from build123d import *

# Parameters (mm, degrees)
SKETCH1_W           = 25
SKETCH1_H           = 135
BOSS_EXTRUDE1_DEPTH = 3.175


with BuildPart() as part:
    # Sketch1 → Boss-Extrude1 (new body)
    with BuildSketch(Plane(origin=(0, 0, 0), x_dir=(1, 0, 0), z_dir=(0, 1, 0))):
        Polygon((67.674333466, 92.651811553), (67.674333466, -62.348188447), (-47.325666534, -62.348188447), (-47.325666534, -27.044565342), (-47.325666534, 92.651811553), align=None)
        with Locations((-6.586624165, 15.039519235)):
            Rectangle(SKETCH1_W, SKETCH1_H, mode=Mode.SUBTRACT)
        with BuildLine():
            Line((-34.586624165, 63.427366475), (-34.586624165, 83.427366475))
            ThreePointArc((-34.586624165, 83.427366475), (-32.086624165, 85.927366475), (-29.586624165, 83.427366475))
            Line((-29.586624165, 83.427366475), (-29.586624165, 63.427366475))
            ThreePointArc((-29.586624165, 63.427366475), (-32.086624165, 60.927366475), (-34.586624165, 63.427366475))
        make_face(mode=Mode.SUBTRACT)
        with BuildLine():
            Line((-34.586624165, 3.427366475), (-34.586624165, 23.427366475))
            ThreePointArc((-34.586624165, 23.427366475), (-32.086624165, 25.927366475), (-29.586624165, 23.427366475))
            Line((-29.586624165, 23.427366475), (-29.586624165, 3.427366475))
            ThreePointArc((-29.586624165, 3.427366475), (-32.086624165, 0.927366475), (-34.586624165, 3.427366475))
        make_face(mode=Mode.SUBTRACT)
        with BuildLine():
            Line((59.674333466, 7.651811553), (59.674333466, 27.651811553))
            ThreePointArc((59.674333466, 27.651811553), (61.674333466, 29.651811553), (63.674333466, 27.651811553))
            Line((63.674333466, 27.651811553), (63.674333466, 7.651811553))
            ThreePointArc((63.674333466, 7.651811553), (61.674333466, 5.651811553), (59.674333466, 7.651811553))
        make_face(mode=Mode.SUBTRACT)
        with BuildLine():
            Line((59.674333466, -40.348188447), (59.674333466, -20.348188447))
            ThreePointArc((59.674333466, -20.348188447), (61.674333466, -18.348188447), (63.674333466, -20.348188447))
            Line((63.674333466, -20.348188447), (63.674333466, -40.348188447))
            ThreePointArc((63.674333466, -40.348188447), (61.674333466, -42.348188447), (59.674333466, -40.348188447))
        make_face(mode=Mode.SUBTRACT)
        with BuildLine():
            Line((41.674333466, 7.651811553), (41.674333466, 27.651811553))
            ThreePointArc((41.674333466, 27.651811553), (39.674333466, 29.651811553), (37.674333466, 27.651811553))
            Line((37.674333466, 27.651811553), (37.674333466, 7.651811553))
            ThreePointArc((37.674333466, 7.651811553), (39.674333466, 5.651811553), (41.674333466, 7.651811553))
        make_face(mode=Mode.SUBTRACT)
        with BuildLine():
            Line((41.674333466, -40.348188447), (41.674333466, -20.348188447))
            ThreePointArc((41.674333466, -20.348188447), (39.674333466, -18.348188447), (37.674333466, -20.348188447))
            Line((37.674333466, -20.348188447), (37.674333466, -40.348188447))
            ThreePointArc((37.674333466, -40.348188447), (39.674333466, -42.348188447), (41.674333466, -40.348188447))
        make_face(mode=Mode.SUBTRACT)
    extrude(amount=BOSS_EXTRUDE1_DEPTH)


solid = part.part
Geometry check sheet. Reference: the model listing, model coordinates, mm. A direction names the side the tool comes from. Round coordinates to 2 decimals unless told otherwise and drop trailing zeros. Loops run counter-clockwise (first coordinate to the right, second up) from the corner with the lowest first, then second, coordinate; pieces in that order, holes last. Notation, with made-up numbers: (-3.5, 47.5) - (26.5, 47.5) arc R12 ccw to (26.5, 58.5) - close; hole circle Ø2 at (28, 62). An arc over 180 degrees is marked (long way). One line per question, with ' | ' between items. Start each with the question number.
1. Scan lines: line 1 (X direction, y = 2.95, z = -76); line 2 (X direction, y = 1.6, z = -14); line 3 (X direction, y = 1.9, z = 26). Record each from-to range of solid material in increasing order. Write a range as [from, to].
2. Tool access check on faces 1 (the face through (63.674, 2, 30)), 2 (the face through (11, 3.175, -16)). Record the directions out of +Z, -Z, +X, -X, +Y, -Y that give a thin tool (end or side, any length) a straight path to the whole face; none if there is none.
3. Cross-section at B-B on x = -7. Record the cut outline in (y, z) (3 decimals).
4. Draft check along X on faces 3 (the face through (11, 2, 62.348)), 4 (the face through (37.674, 2, -18)), 5 (the face through (-47.326, 2, -16)). Enter one of: released by +X, released by -X, zero draft, split by the parting line, or undercut.
5. Cross-section at D-D on y = 1.35. State how many separate pieces and enclosed holes the cut face has, then the cut area to 3 significant figures.
6. Cross-section at A-A on z = -69. Record the cut outline in (x, y) (3 decimals), then the cut area to 3 significant figures.
7. Cross-section at C-C on z = 30.5. Record the cut outline in (x, y) (3 decimals).
Taken from the geometry:
1) line 1: [-47.33, -34.59], [-29.59, -19.09], [5.91, 67.67] | line 2: [-47.33, -34.59], [-29.59, -19.09], [5.91, 37.67], [41.67, 59.67], [63.67, 67.67] | line 3: [-47.33, -19.09], [5.91, 37.67], [41.67, 59.67], [63.67, 67.67]
2) face 1: +Y, -Y | face 2: +Z, -Z, +X, -X, +Y
3) outline: (0, -92.652) - (3.175, -92.652) - (3.175, -82.54) - (0, -82.54) - close; (0, 52.46) - (3.175, 52.46) - (3.175, 62.348) - (0, 62.348) - close
4) face 3: zero draft | face 4: undercut | face 5: released by -X
5) separate pieces: 1 | enclosed holes: 7 | area: 13,800 mm²
6) outline: (-47.326, 0) - (-34.587, 0) - (-34.587, 3.175) - (-47.326, 3.175) - close; (-29.587, 0) - (-19.087, 0) - (-19.087, 3.175) - (-29.587, 3.175) - close; (5.913, 0) - (67.674, 0) - (67.674, 3.175) - (5.913, 3.175) - close | area: 270 mm²
7) outline: (-47.326, 0) - (-19.087, 0) - (-19.087, 3.175) - (-47.326, 3.175) - close; (5.913, 0) - (37.674, 0) - (37.674, 3.175) - (5.913, 3.175) - close; (41.674, 0) - (59.674, 0) - (59.674, 3.175) - (41.674, 3.175) - close; (63.674, 0) - (67.674, 0) - (67.674, 3.175) - (63.674, 3.175) - close
